The model under review builds one solid part; all positions refer to its coordinate system, in mm. A direction names the side the tool comes from. Round coordinates to 2 decimals unless told otherwise and drop trailing zeros. Loops run counter-clockwise (first coordinate to the right, second up) from the corner with the lowest first, then second, coordinate; pieces in that order, holes last. Notation, with made-up numbers: M 80,47.25 L 139,47.25 A14 cw 139,60.25 Z; hole C 60.5,-38.75 d9. An arc over 180 degrees is marked long. Use a Markdown table: item, result. Add a question column.
```python
from build123d import *

# Parameters (mm, degrees)
SKETCH1_R           = 5.65
BOSS_EXTRUDE1_DEPTH = 12
SKETCH2_R           = 5.65
BOSS_EXTRUDE2_DEPTH = 14.74
SKETCH3_R           = 5.65
BOSS_EXTRUDE3_DEPTH = 14
SKETCH5_R           = 4.25
SKETCH5_R_2         = 2.175
BOSS_EXTRUDE4_DEPTH = 5.2
SKETCH5_2_R         = 2.175
CUT_EXTRUDE1_DEPTH  = 42.988958203


with BuildPart() as part:
    # Sketch1 → Boss-Extrude1 (new body)
    # profile 1 of 12: a face of its own
    with BuildSketch(Plane.XY):
        Circle(SKETCH1_R)
        with BuildLine():
            ThreePointArc((-0.81964124, -3.557591308), (-1.028546403, -3.50290736), (-1.233852984, -3.435967766))
            ThreePointArc((-1.233852984, -3.435967766), (-1.973766094, -3.071239991), (-2.612905161, -2.549704746))
            ThreePointArc((-2.612905161, -2.549704746), (-2.759082994, -2.390759024), (-2.895607604, -2.223448736))
            ThreePointArc((-2.895607604, -2.223448736), (-3.320875399, -1.516592978), (-3.576590156, -0.732304943))
            ThreePointArc((-3.576590156, -0.732304943), (-3.613630229, -0.519561589), (-3.638027269, -0.305000442))
            ThreePointArc((-3.638027269, -0.305000442), (-3.613630229, 0.519561589), (-3.404733048, 1.317596505))
            ThreePointArc((-3.404733048, 1.317596505), (-3.320875399, 1.516592978), (-3.225398981, 1.710283337))
            ThreePointArc((-3.225398981, 1.710283337), (-2.759082994, 2.390759024), (-2.151897253, 2.949170373))
            ThreePointArc((-2.151897253, 2.949170373), (-1.973766094, 3.071239991), (-1.788729306, 3.182564241))
            ThreePointArc((-1.788729306, 3.182564241), (-1.028546403, 3.50290736), (-0.215849285, 3.644403485))
            ThreePointArc((-0.215849285, 3.644403485), (-0.107971873, 3.649193027), (0, 3.650790007))
            ThreePointArc((0, 3.650790007), (0.107971873, 3.649193027), (0.215849285, 3.644403485))
            ThreePointArc((0.215849285, 3.644403485), (1.028546403, 3.50290736), (1.788729306, 3.182564241))
            ThreePointArc((1.788729306, 3.182564241), (1.973766094, 3.071239991), (2.151897253, 2.949170373))
            ThreePointArc((2.151897253, 2.949170373), (2.759082994, 2.390759024), (3.225398981, 1.710283337))
            ThreePointArc((3.225398981, 1.710283337), (3.320875399, 1.516592978), (3.404733048, 1.317596505))
            ThreePointArc((3.404733048, 1.317596505), (3.588748603, 0.670187395), (3.650790007, 0))
            ThreePointArc((3.650790007, 0), (3.647597927, -0.152633677), (3.638027269, -0.305000442))
            ThreePointArc((3.638027269, -0.305000442), (3.613630229, -0.519561589), (3.576590156, -0.732304943))
            ThreePointArc((3.576590156, -0.732304943), (3.320875399, -1.516592978), (2.895607604, -2.223448736))
            ThreePointArc((2.895607604, -2.223448736), (2.759082994, -2.390759024), (2.612905161, -2.549704746))
            ThreePointArc((2.612905161, -2.549704746), (1.973766094, -3.071239991), (1.233852984, -3.435967766))
            ThreePointArc((1.233852984, -3.435967766), (1.028546403, -3.50290736), (0.81964124, -3.557591308))
            ThreePointArc((0.81964124, -3.557591308), (0, -3.650790007), (-0.81964124, -3.557591308))
        make_face(mode=Mode.SUBTRACT)
    # profile 2 of 12: a face of its own
    with BuildSketch(Plane.XY):
        with BuildLine():
            ThreePointArc((-2.151897253, 2.949170373), (-2.759082994, 2.390759024), (-3.225398981, 1.710283337))
            ThreePointArc((-3.225398981, 1.710283337), (-2.902782795, 1.721509121), (-2.585426091, 1.662416447))
            ThreePointArc((-2.585426091, 1.662416447), (-2.562741672, 1.6561643), (-2.539777266, 1.651035136))
            ThreePointArc((-2.539777266, 1.651035136), (-2.085465777, 1.807066382), (-1.99567797, 2.278959198))
            ThreePointArc((-1.99567797, 2.278959198), (-2.004023102, 2.300959902), (-2.013439941, 2.322523654))
            ThreePointArc((-2.013439941, 2.322523654), (-2.117095704, 2.628240359), (-2.151897253, 2.949170373))
        make_face()
    # profile 3 of 12: a face of its own
    with BuildSketch(Plane.XY):
        with BuildLine():
            ThreePointArc((-0.215849285, 3.644403485), (-1.028546403, 3.50290736), (-1.788729306, 3.182564241))
            ThreePointArc((-1.788729306, 3.182564241), (-1.511258183, 3.017588493), (-1.276228646, 2.796300584))
            ThreePointArc((-1.276228646, 2.796300584), (-1.260525464, 2.77877682), (-1.243979612, 2.762046398))
            ThreePointArc((-1.243979612, 2.762046398), (-0.777431606, 2.6476889), (-0.446772779, 2.996127445))
            ThreePointArc((-0.446772779, 2.996127445), (-0.441898672, 3.019147334), (-0.438162377, 3.042379044))
            ThreePointArc((-0.438162377, 3.042379044), (-0.360080224, 3.355604839), (-0.215849285, 3.644403485))
        make_face()
    # profile 4 of 12: a face of its own
    with BuildSketch(Plane.XY):
        with BuildLine():
            ThreePointArc((1.788729306, 3.182564241), (1.028546403, 3.50290736), (0.215849285, 3.644403485))
            ThreePointArc((0.215849285, 3.644403485), (0.360080224, 3.355604839), (0.438162377, 3.042379044))
            ThreePointArc((0.438162377, 3.042379044), (0.441898672, 3.019147334), (0.446772779, 2.996127445))
            ThreePointArc((0.446772779, 2.996127445), (0.777431606, 2.6476889), (1.243979612, 2.762046398))
            ThreePointArc((1.243979612, 2.762046398), (1.260525464, 2.77877682), (1.276228646, 2.796300584))
            ThreePointArc((1.276228646, 2.796300584), (1.511258183, 3.017588493), (1.788729306, 3.182564241))
        make_face()
    # profile 5 of 12: a face of its own
    with BuildSketch(Plane.XY):
        with BuildLine():
            ThreePointArc((2.585426091, 1.662416447), (2.902782795, 1.721509121), (3.225398981, 1.710283337))
            ThreePointArc((3.225398981, 1.710283337), (2.759082994, 2.390759024), (2.151897253, 2.949170373))
            ThreePointArc((2.151897253, 2.949170373), (2.117095704, 2.628240359), (2.013439941, 2.322523654))
            ThreePointArc((2.013439941, 2.322523654), (2.004023102, 2.300959902), (1.99567797, 2.278959198))
            ThreePointArc((1.99567797, 2.278959198), (2.085465777, 1.807066382), (2.539777266, 1.651035136))
            ThreePointArc((2.539777266, 1.651035136), (2.562741672, 1.6561643), (2.585426091, 1.662416447))
        make_face()
    # profile 6 of 12: a face of its own
    with BuildSketch(Plane.XY):
        with BuildLine():
            ThreePointArc((3.07376902, 0.000726834), (3.372694379, -0.121137234), (3.638027269, -0.305000442))
            ThreePointArc((3.638027269, -0.305000442), (3.647597927, -0.152633677), (3.650790007, 0))
            ThreePointArc((3.650790007, 0), (3.588748603, 0.670187395), (3.404733048, 1.317596505))
            ThreePointArc((3.404733048, 1.317596505), (3.201948257, 1.066428135), (2.94946455, 0.865283413))
            ThreePointArc((2.94946455, 0.865283413), (2.929884357, 0.852233959), (2.910969506, 0.838237507))
            ThreePointArc((2.910969506, 0.838237507), (2.731379298, 0.392713056), (3.029213584, 0.015831883))
            ThreePointArc((3.029213584, 0.015831883), (3.051305506, 0.007731316), (3.07376902, 0.000726834))
        make_face()
    # profile 7 of 12: a face of its own
    with BuildSketch(Plane.XY):
        with BuildLine():
            ThreePointArc((2.586212003, -1.661193544), (2.771799329, -1.925323372), (2.895607604, -2.223448736))
            ThreePointArc((2.895607604, -2.223448736), (3.320875399, -1.516592978), (3.576590156, -0.732304943))
            ThreePointArc((3.576590156, -0.732304943), (3.270204862, -0.833967486), (2.949055004, -0.866678197))
            ThreePointArc((2.949055004, -0.866678197), (2.92552803, -0.867070245), (2.902048792, -0.868618669))
            ThreePointArc((2.902048792, -0.868618669), (2.510099192, -1.146323891), (2.556895991, -1.62439788))
            ThreePointArc((2.556895991, -1.62439788), (2.571101401, -1.643156306), (2.586212003, -1.661193544))
        make_face()
    # profile 8 of 12: a face of its own
    with BuildSketch(Plane.XY):
        with BuildLine():
            ThreePointArc((1.277550948, -2.79569671), (1.290877576, -3.118232944), (1.233852984, -3.435967766))
            ThreePointArc((1.233852984, -3.435967766), (1.973766094, -3.071239991), (2.612905161, -2.549704746))
            ThreePointArc((2.612905161, -2.549704746), (2.300194531, -2.469584323), (2.012341335, -2.323475602))
            ThreePointArc((2.012341335, -2.323475602), (1.992337228, -2.311085771), (1.971748095, -2.299694554))
            ThreePointArc((1.971748095, -2.299694554), (1.491880328, -2.321411101), (1.272781988, -2.748892795))
            ThreePointArc((1.272781988, -2.748892795), (1.274590768, -2.772353412), (1.277550948, -2.79569671))
        make_face()
    # profile 9 of 12: a face of its own
    with BuildSketch(Plane.XY):
        with BuildLine():
            ThreePointArc((-0.436723505, -3.042585922), (-0.599888686, -3.321125588), (-0.81964124, -3.557591308))
            ThreePointArc((-0.81964124, -3.557591308), (0, -3.650790007), (0.81964124, -3.557591308))
            ThreePointArc((0.81964124, -3.557591308), (0.599888686, -3.321125588), (0.436723505, -3.042585922))
            ThreePointArc((0.436723505, -3.042585922), (0.426593428, -3.021347897), (0.415431304, -3.00063367))
            ThreePointArc((0.415431304, -3.00063367), (0, -2.75946669), (-0.415431304, -3.000633669))
            ThreePointArc((-0.415431304, -3.000633669), (-0.426593428, -3.021347896), (-0.436723505, -3.042585922))
        make_face()
    # profile 10 of 12: a face of its own
    with BuildSketch(Plane.XY):
        with BuildLine():
            ThreePointArc((-1.233852984, -3.435967766), (-1.290877576, -3.118232944), (-1.277550949, -2.79569671))
            ThreePointArc((-1.277550949, -2.79569671), (-1.274590768, -2.772353411), (-1.272781988, -2.748892794))
            ThreePointArc((-1.272781988, -2.748892794), (-1.491880327, -2.321411102), (-1.971748091, -2.299694555))
            ThreePointArc((-1.971748091, -2.299694555), (-1.992337225, -2.311085772), (-2.012341332, -2.323475603))
            ThreePointArc((-2.012341332, -2.323475603), (-2.300194529, -2.469584324), (-2.612905161, -2.549704746))
            ThreePointArc((-2.612905161, -2.549704746), (-1.973766094, -3.071239991), (-1.233852984, -3.435967766))
        make_face()
    # profile 11 of 12: a face of its own
    with BuildSketch(Plane.XY):
        with BuildLine():
            ThreePointArc((-3.576590156, -0.732304943), (-3.320875399, -1.516592978), (-2.895607604, -2.223448736))
            ThreePointArc((-2.895607604, -2.223448736), (-2.771799329, -1.925323372), (-2.586212003, -1.661193544))
            ThreePointArc((-2.586212003, -1.661193544), (-2.571101401, -1.643156306), (-2.556895991, -1.62439788))
            ThreePointArc((-2.556895991, -1.62439788), (-2.510099192, -1.146323891), (-2.902048792, -0.868618669))
            ThreePointArc((-2.902048792, -0.868618669), (-2.92552803, -0.867070245), (-2.949055004, -0.866678197))
            ThreePointArc((-2.949055004, -0.866678197), (-3.270204862, -0.833967486), (-3.576590156, -0.732304943))
        make_face()
    # profile 12 of 12: a face of its own
    with BuildSketch(Plane.XY):
        with BuildLine():
            ThreePointArc((-3.404733048, 1.317596505), (-3.613630229, 0.519561589), (-3.638027269, -0.305000442))
            ThreePointArc((-3.638027269, -0.305000442), (-3.372694379, -0.121137234), (-3.07376902, 0.000726834))
            ThreePointArc((-3.07376902, 0.000726834), (-3.051305506, 0.007731316), (-3.029213584, 0.015831883))
            ThreePointArc((-3.029213584, 0.015831883), (-2.731379298, 0.392713056), (-2.910969506, 0.838237507))
            ThreePointArc((-2.910969506, 0.838237507), (-2.929884357, 0.852233959), (-2.94946455, 0.865283413))
            ThreePointArc((-2.94946455, 0.865283413), (-3.201948257, 1.066428135), (-3.404733048, 1.317596505))
        make_face()
    extrude(amount=BOSS_EXTRUDE1_DEPTH)

    # Sketch2 → Boss-Extrude2 (add)
    with BuildSketch(Plane.XY.offset(12)):
        Circle(SKETCH2_R)
    extrude(amount=BOSS_EXTRUDE2_DEPTH)

    # Sketch3 → Boss-Extrude3 (add)
    with BuildSketch(Plane.XY.offset(26.74)):
        Circle(SKETCH3_R)
        with BuildLine():
            Line((-1.74642492, 2.8), (1.74642492, 2.8))
            ThreePointArc((1.74642492, 2.8), (0, -3.3), (-1.74642492, 2.8))
        make_face(mode=Mode.SUBTRACT)
    extrude(amount=BOSS_EXTRUDE3_DEPTH)

    # Sketch5 → Boss-Extrude4 (add)
    with BuildSketch(Plane.XZ.offset(-2.8)):
        with Locations(Location((0, 29.915, 0), (0, 0, 270))):
            Circle(SKETCH5_R)
        with Locations(Location((0, 29.915, 0), (0, 0, 270))):
            Circle(SKETCH5_R_2, mode=Mode.SUBTRACT)
    extrude(amount=-BOSS_EXTRUDE4_DEPTH)

    # Sketch5<2> → Cut-Extrude1 (cut, through all)
    with BuildSketch(Plane.XZ.offset(-2.8)):
        with Locations(Location((0, 29.915, 0), (0, 0, 270))):
            Circle(SKETCH5_2_R)
    extrude(amount=-CUT_EXTRUDE1_DEPTH, mode=Mode.SUBTRACT)


solid = part.part
```
(1) Consider section D-D, the plane z = 30. Give the boundary of the cut face in (x, y).
(2) Consider section B-B, the plane y = 6.25. Give the boundary of the cut face in (x, z) (3 decimals).
(3) Insertion check: pin 1 Ø1.5 at (y, z) = (5.5, 33.5) entering from +X; pin 2 Ø1.7 at (x, z) = (0.5, 38) entering from -Y; pin 3 Ø1.8 at (x, y) = (-0.5, 1) entering from +Z; pin 4 Ø3.5 at (x, y) = (0, 0) entering from -Z. Each pin has a flat end and moves straight along its axis. Give the tip position at first contact, or say it passes through.
(4) To check wall thickness, follow probe 1 along Z at (x, y) = (0, 4.45); probe 2 along Z at (x, y) = (0, 6.25) (3 decimals); probe 3 along X at (y, z) = (-0.25, 34). State the ranges of each line that lie inside material, in increasing order.
(5) Draft analysis for pull direction X (two halves, no side actions). For faces 1 (the face through (0, 2.8, 36)), 2 (the face through (-1.225, -5.516, 20.085)), 3 (the face through (-2, 8, 28)), state which applies: released by +X, released by -X, zero draft, split by the parting line, or undercut.
(6) Consider section C-C, the plane z = 23. Give the boundary of the cut face in (x, y), then the cut area to 3 significant figures.
(7) Consider section A-A, the plane z = 37.5. Give the boundary of the cut face in (x, y).
(8) For faces 4 (the face through (0, 0, 12)), 5 (the face through (0, 2.8, 27)), 6 (the face through (2.87, 6.31, 33.05)), list the 3-axis set-ups (+Z, -Z, +X, -X, +Y, -Y) from which the entire face can be reached by the end or side of a thin tool; tool diameter is ignored.
Found:
| question | item | result |
|---|---|---|
| 1 | outline | M -4.25,3.72 A5.65 ccw long 4.25,3.72 L 4.25,8 L 2.17,8 L 2.17,2.8 L 1.75,2.8 A3.3 cw long -1.75,2.8 L -2.17,2.8 L -2.17,8 L -4.25,8 Z |
| 2 | outline | C 0,29.915 d8.5; hole C 0,29.915 d4.35 |
| 3 | pin 1 | stops at x = 3.17 |
| 3 | pin 2 | stops at y = -5.65 |
| 3 | pin 3 | stops at z = 26.74 |
| 3 | pin 4 | stops at z = 12 |
| 4 | probe 1 | z = 0 to 27.74, 32.09 to 40.74 |
| 4 | probe 2 | z = 25.665 to 27.74, 32.09 to 34.165 |
| 4 | probe 3 | x = -5.64 to -3.29, 3.29 to 5.64 |
| 5 | face 1 | undercut |
| 5 | face 2 | split by the parting line |
| 5 | face 3 | zero draft |
| 6 | outline | C 0,0 d11.3 |
| 6 | area | 100 mm^2 |
| 7 | outline | C 0,0 d11.3; hole M -1.75,2.8 A3.3 ccw long 1.75,2.8 Z |
| 8 | face 4 | -Z |
| 8 | face 5 | +Z |
| 8 | face 6 | +Y |
